```python
from build123d import *

# Parameters (mm, degrees)
SKETCH1_R           = 5
BOSS_EXTRUDE1_DEPTH = 17
SKETCH2_R           = 10.5
CUT_EXTRUDE1_DEPTH  = 64
CUT_EXTRUDE2_DEPTH  = 8


with BuildPart() as part:
    # Sketch1 → Boss-Extrude1 (new body)
    with BuildSketch(Plane(origin=(0, 0, 0), x_dir=(1, 0, 0), z_dir=(0, 1, 0))):
        with BuildLine():
            Line((-38, 0), (-38, 35))
            ThreePointArc((-38, 35), (-47, 44), (-56, 35))
            Line((-56, 35), (-56, 0))
            ThreePointArc((-56, 0), (-47, -9), (-38, 0))
        make_face()
        with Locations(Location((-47, 35, 0), (0, 0, 270))):
            Circle(SKETCH1_R, mode=Mode.SUBTRACT)
        with Locations(Location((-47, 0, 0), (0, 0, 270))):
            Circle(SKETCH1_R, mode=Mode.SUBTRACT)
    extrude(amount=BOSS_EXTRUDE1_DEPTH)

    # Sketch2 → Cut-Extrude1 (cut)
    with BuildSketch(Plane(origin=(0, 0, 0), x_dir=(0, 0, -1), z_dir=(1, 0, 0))):
        with Locations((17.5, 22)):
            Circle(SKETCH2_R)
    extrude(amount=-CUT_EXTRUDE1_DEPTH, mode=Mode.SUBTRACT)

    # Sketch3 → Cut-Extrude2 (cut)
    with BuildSketch(Plane.XZ):
        with BuildLine():
            Line((-52, -7.483314774), (-52, -27.516685226))
            ThreePointArc((-52, -27.516685226), (-47, -26), (-42, -27.516685226))
            Line((-42, -27.516685226), (-42, -7.483314774))
            ThreePointArc((-42, -7.483314774), (-47, -9), (-52, -7.483314774))
        make_face()
    extrude(amount=-CUT_EXTRUDE2_DEPTH, mode=Mode.SUBTRACT)


solid = part.part
```
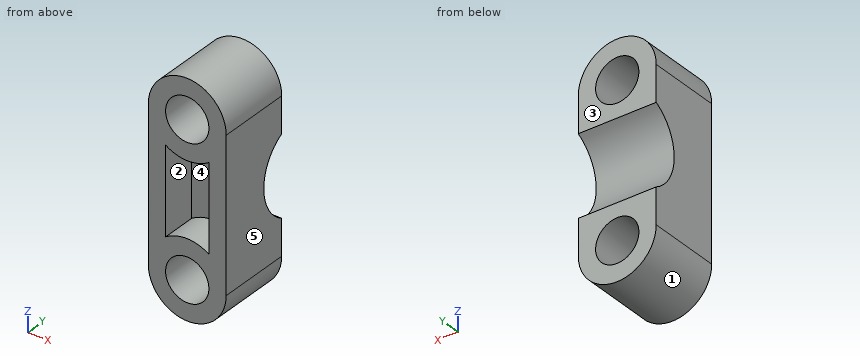
Source: CAD feature listing. Evaluate the final solid. Frame: model axes, mm. Face numbers are marked on the shaded views. A direction names the side the tool comes from. Coordinates: 2 decimals unless noted, no trailing zeros. Order: outer loops, then holes, each group sorted by start corner. A loop starts at its lowest first (then second) coordinate and runs counter-clockwise, first axis right, second up. Notation, with made-up numbers: (81.5, 0) - (134.5, 0) arc R24 cw to (134.5, 24) - close; hole circle Ø3 at (62, -26.75). An arc over 180 degrees is marked (long way). One line per item, written item: value.
1) Ray query, line 1 (X direction, y = 12.25, z = 0); line 2 (Z direction, x = -46.5, y = 10.25); line 3 (Z direction, x = -49, y = 9.5). Return the intervals inside material, ascending. Write a range as [from, to].
Computed values:
line 1: x = [-56, -52], [-42, -38]
line 2: z = [-43.99, -39.97], [-30.03, -4.97], [4.97, 8.99]
line 3: z = [-43.77, -39.58], [-30.42, -4.58], [4.58, 8.77]
2) Contact query for flat-ended pins moving along their axis: pin 1 (8 mm diameter, centred on x = -46.5, z = -15.5, fed in from -Y); pin 2 (5 mm diameter, centred on x = -54, y = 5, fed in from -Z). Output: stop coordinate, or through.
Computed values:
pin 1: stops at y = 8
pin 2: stops at z = -42.79
3) Cut plane D-D on y = 15.75. Output: boundary loops of the cut face in (x, z).
Computed values:
outline: (-56, -35) arc R9 ccw to (-38, -35) - (-38, -25.94) - (-56, -25.94) - close; (-56, -9.06) - (-38, -9.06) - (-38, 0) arc R9 ccw to (-56, 0) - close; hole circle Ø10 at (-47, -35); hole circle Ø10 at (-47, 0)
4) Cut plane B-B on z = 3.5. Output: boundary loops of the cut face in (x, y).
Computed values:
outline: (-55.29, 0) - (-50.57, 0) - (-50.57, 17) - (-55.29, 17) - close; (-43.43, 0) - (-38.71, 0) - (-38.71, 17) - (-43.43, 17) - close
5) Mould query, pull axis Z, two halves, no side actions, for the marked faces 1, 2 and 3. Classes: released by +Z, released by -Z, zero draft, split by the parting line, or undercut.
Computed values:
face 1: released by -Z
face 2: undercut
face 3: zero draft
6) Reachability of the marked faces 4 and 5 from +Z, -Z, +X, -X, +Y, -Y: full face, straight path, thin tool, end or side. Return the list, or none.
Computed values:
face 4: -Y
face 5: +Z, -Z, +X, +Y, -Y
7) Cut plane C-C on x = -47. Output: boundary loops of the cut face in (y, z), plus the area to 3 significant figures.
Computed values:
outline: (0, -44) - (17, -44) - (17, -40) - (0, -40) - close; (0, -30) - (17, -30) - (17, -26.73) arc R10.5 cw to (17, -8.27) - (17, -5) - (0, -5) - (0, -9) - (8, -9) - (8, -26) - (0, -26) - close; (0, 5) - (17, 5) - (17, 9) - (0, 9) - close
area: 353 mm^2
8) Cut plane A-A on y = 3.75. Output: boundary loops of the cut face in (x, z), plus the area to 3 significant figures.
Computed values:
outline: (-56, -35) arc R9 ccw to (-38, -35) - (-38, 0) arc R9 ccw to (-56, 0) - close; hole circle Ø10 at (-47, -35); hole (-52, -27.52) arc R9 cw to (-42, -27.52) - (-42, -7.48) arc R9 cw to (-52, -7.48) - close; hole circle Ø10 at (-47, 0)
area: 548 mm^2
